Part model, mm, in its own coordinate system. A direction names the side the tool comes from. Coordinates: 2 decimals unless noted, no trailing zeros. Loops run counter-clockwise (first coordinate to the right, second up) from the corner with the lowest first, then second, coordinate; pieces in that order, holes last. Notation, with made-up numbers: M 51,-9 L 81,-9 A29 ccw 81,23 Z; hole C -2.5,82 d4. An arc over 180 degrees is marked long. Answer as a JSON object with one key per item and string values. Group by question number.
1. 3-axis set-ups, long thin cutter, end or side, ignore diameter. For faces 1 (the face through (32.5, 13, 41)), 2 (the face through (1, 30, 0.5)), 3 (the face through (68, 29, -28)): which of +Z, -Z, +X, -X, +Y, -Y reach the whole face in a straight line?
2. Saw through at B-B on y = 22. Write the cut outline in (x, z), then the cut area to 3 significant figures.
3. Saw through at D-D on z = 35. Write the cut outline in (x, y).
4. Drill centre lines: L1, parallel to Z at x = -29, y = 2.75; L2, parallel to X at y = 4.5, z = 35; L3, parallel to X at y = 21.5, z = -39. Where is each one in solid material? Low to high.
5. Mould opens along Z. For faces 4 (the face through (-1, 22, -42.5)), 5 (the face through (-28.82, 4.44, 33.61)), 6 (the face through (70, 22, -1)), 7 (the face through (-69, 29, -13)) say: released by +Z, released by -Z, zero draft, split by the parting line, or undercut.
6. Drop flat-ended pins along their axis: pin 1 Ø2 at (x, z) = (29, 35) entering from +Y; pin 2 Ø2 at (x, z) = (33, 4) entering from +Y; pin 3 Ø10 at (x, z) = (6, 3.5) entering from +Y. Give the stop position or say it passes through.
Autodesk Inventor part; units mm, degrees
ref_plane "YZ Plane" through (0, 0, 0) normal (1, 0, 0) x (0, 1, 0)
ref_plane "XZ Plane" through (0, 0, 0) normal (0, 1, 0) x (-1, 0, 0)
ref_plane "XY Plane" through (0, 0, 0) normal (0, 0, 1) x (1, 0, 0)
sketch "Sketch1" plane through (0, 0, 0) normal (0, 1, 0) x (-1, 0, 0)
  line L0 (70, -42.5) -> (-70, -42.5)
  line L1 (-70, -42.5) -> (-70, 42.5)
  line L2 (-70, 42.5) -> (70, 42.5)
  line L3 (70, 42.5) -> (70, -42.5)
  line L4 (70, -42.5) -> (-70, 42.5) construction
  line L5 (-70, -42.5) -> (70, 42.5) construction
  point P0 (0, 0)
  dimension "d0" = 140
  dimension "d1" = 85
extrude "Outer-Shell" add sketch "Sketch1" along normal blind 45
shell "Shell1" thickness 3 removed faces 1 at (-23.3333, 45, -14.1667)
sketch "Sketch2" plane through (-67, 3, 39.5) normal (0, 1, 0) x (1, 0, 0)
  line L0 (0, 79) -> (134, 79)
  line L1 (134, 79) -> (134, 39)
  line L2 (134, 39) -> (0, 39)
  line L3 (0, 39) -> (0, 79)
  line L4 (0, 79) -> (134, 39) construction
  line L5 (134, 79) -> (0, 39) construction
  line L6 (134, 0) -> (134, 79)
  line L7 (0, 79) -> (134, 79)
  line L8 (134, 79) -> (0, 79)
  line L9 (0, 79) -> (0, 0)
  point P0 (67, 39.5)
  point P1 (67, 59)
  dimension "d5" = 40
extrude "Battery_Holder" add sketch "Sketch2" along normal blind 32
sketch "Sketch3" plane through (-67, 3, -39.5) normal (1, 0, 0) x (0, 0, -1)
  circle A0 centre (-20, 22) radius 20
  line L0 (-79, 42) -> (0, 42)
  line L1 (0, 0) -> (0, 42)
  point P0 (-39.5, -3)
  dimension "d8" = 40
  dimension "d9" = 20
extrude "Battery_Cutout" cut sketch "Sketch3" along normal up to surface (134 mm away) contours A0
sketch "Sketch4" plane through (-70, 0, -42.5) normal (-1, 0, 0) x (0, 0, 1)
  line L0 (14.5, 45) -> (29.5, 45)
  line L1 (29.5, 45) -> (29.5, 13)
  line L2 (29.5, 13) -> (14.5, 13)
  line L3 (14.5, 13) -> (14.5, 45)
  line L4 (0, 0) -> (0, 45)
  line L5 (0, 45) -> (85, 45)
  point P0 (42.5, 0)
  dimension "d15" = 15
  dimension "d16" = 32
  dimension "d17" = 14.5
extrude "Voltmeter_Cutouts" cut sketch "Sketch4" along normal through all both and the other way through all
sketch "Sketch5" plane through (0, 0, 0) normal (0, 1, 0) x (-1, 0, 0)
  line L0 (32, 10.5) -> (-32, 10.5)
  line L1 (-32, 10.5) -> (-32, 40.5)
  line L2 (-32, 40.5) -> (32, 40.5)
  line L3 (32, 40.5) -> (32, 10.5)
  line L4 (70, -13) -> (70, 42.5)
  line L5 (32, 40.5) -> (-32, 40.5)
  line L6 (-32, 40.5) -> (-32, 10.5)
  line L7 (-32, 10.5) -> (32, 10.5)
  line L8 (32, 10.5) -> (32, 40.5)
  line L9 (32, 40.5) -> (-32, 10.5) construction
  line L10 (-32, 40.5) -> (32, 10.5) construction
  point P0 (0, 0)
  point P1 (0, 25.5)
  point P2 (0, 25.5)
  dimension "d21" = 10.5
  dimension "d22" = 30
  dimension "d23" = 64
extrude "Controller_Stand" add sketch "Sketch5" along normal blind 9
sketch "Sketch6" plane through (-70, 0, 42.5) normal (0, 0, 1) x (1, 0, 0)
  line L0 (37.5, 17) -> (102.5, 17)
  line L1 (102.5, 17) -> (102.5, 9)
  line L2 (102.5, 9) -> (37.5, 9)
  line L3 (37.5, 9) -> (37.5, 17)
  line L4 (37.5, 17) -> (102.5, 9) construction
  line L5 (102.5, 17) -> (37.5, 9) construction
  line L6 (0, 0) -> (140, 0)
  point P0 (70, 0)
  point P1 (70, 13)
  dimension "d28" = 65
  dimension "d29" = 8
  dimension "d30" = 9
extrude "USB_Access" cut sketch "Sketch6" against normal up to next
sketch "Sketch7" plane through (0, 0, 0) normal (0, 1, 0) x (-1, 0, 0)
  line L0 (29, 12) -> (-29, 12) construction
  line L1 (-29, 12) -> (-29, 35) construction
  line L2 (-29, 35) -> (29, 35) construction
  line L3 (29, 35) -> (29, 12) construction
  line L4 (29, 12) -> (-29, 35) construction
  line L5 (-29, 12) -> (29, 35) construction
  circle A0 centre (29, 12) radius 1.4
  circle A1 centre (-29, 12) radius 1.4
  circle A2 centre (-29, 35) radius 1.4
  circle A3 centre (29, 35) radius 1.4
  point P0 (0, 0)
  point P1 (0, 23.5)
  point P2 (0, 23.5)
  dimension "d33" = 23
  dimension "d34" = 58
  dimension "d35" = 12
  dimension "d36" = 2.8
extrude "M3_Mount_Holes" cut sketch "Sketch7" along normal through all both and the other way through all
equation "\"d1\" = 0.607143 * d0"
equation "\"d2\" = 0.321429 * d0"
equation "\"d4\" = 0.0214286 * d0"
equation "\"d5\" = 0.285714 * d0"
equation "\"d6\" = 0.8 * d5"
equation "\"d8\" = d5"
equation "\"d9\" = 0.142857 * d0"
equation "\"d10\" = d5"
equation "\"d15\" = 0.107143 * d0"
equation "\"d16\" = 0.228571 * d0"
equation "\"d17\" = 0.103571 * d0"
equation "\"d22\" = 0.214286 * d0"
equation "\"d23\" = 2.13333 * d22"
equation "\"d24\" = 0.3 * d22"
equation "\"d28\" = 2.16667 * d22"
equation "\"d29\" = 0.266667 * d22"
equation "\"d30\" = 0.3 * d22"
equation "\"d31\" = 0.3 * d22"
equation "\"d33\" = 0.164286 * d0"
equation "\"d34\" = 0.414286 * d0"
equation "\"d36\" = 0.02 * d0"
properties part number "Bottom-Shell" material "ABS Plastic"
Outcome:
{
 "1": {"face 1": "+Z", "face 2": "+Y", "face 3": "+X, -X, +Y"},
 "2": {"outline": "M -70,-42.5 L 70,-42.5 L 70,-28 L 67,-28 L 67,-39.27 L -67,-39.27 L -67,-28 L -70,-28 Z; M -70,-13 L -67,-13 L -67,0.27 L 67,0.27 L 67,-13 L 70,-13 L 70,42.5 L -70,42.5 Z; hole M -67,0.5 L 67,0.5 L 67,39.5 L -67,39.5 Z", "area": "1,280 mm²"},
 "3": {"outline": "M -70,0 L -30.4,0 L -30.4,9 L -32,9 L -32,3 L -67,3 L -67,45 L -70,45 Z; M -27.6,0 L 27.6,0 L 27.6,9 L -27.6,9 Z; M 30.4,0 L 70,0 L 70,45 L 67,45 L 67,3 L 32,3 L 32,9 L 30.4,9 Z"},
 "4": {"L1": "z = -42.5 to 10.6, 13.4 to 33.6, 36.4 to 42.5", "L2": "x = -70 to -67, -32 to -30.4, -27.6 to 27.6, 30.4 to 32, 67 to 70", "L3": "x = -70 to -67, 67 to 70"},
 "5": {"face 4": "released by -Z", "face 5": "undercut", "face 6": "zero draft", "face 7": "undercut"},
 "6": {"pin 1": "passes through", "pin 2": "stops at y = 3", "pin 3": "stops at y = 35"}
}
